from build123d import *

# Parameters (mm, degrees)
SKETCH_1_R        = 3
SKETCH_1_R_2      = 1.5
EXTRUDE_1_DEPTH   = 1.2
EXTRUDE_1_2_DEPTH = 1.2
EXTRUDE_2_DEPTH   = 1.2
FILLET_1_R        = 1


with BuildPart() as part:
    # Sketch 1 → Extrude 1 (new body)
    with BuildSketch(Plane.XY):
        with Locations((-4.672939719, 0.001012373)):
            Circle(SKETCH_1_R)
        with Locations((-4.672939719, 0.001012373)):
            Circle(SKETCH_1_R_2, mode=Mode.SUBTRACT)
    extrude(amount=EXTRUDE_1_DEPTH)



with BuildPart() as body_2:
    # Sketch 1 → Extrude 1 2 (new body)
    with BuildSketch(Plane.XY):
        with Locations((4.672939719, -0.001012373)):
            Circle(SKETCH_1_R)
        with Locations((4.672939719, -0.001012373)):
            Circle(SKETCH_1_R_2, mode=Mode.SUBTRACT)
    extrude(amount=EXTRUDE_1_2_DEPTH)


with BuildPart() as part_1:
    add(part.part)

    add(body_2.part)  # Extrude 2 merges body 2
    # Sketch 2 → Extrude 2 (add)
    with BuildSketch(Plane.XY.offset(1.2)):
        Polygon((-4.672103484, 3.001012257), (4.673403359, 2.998987591), (1.672939725, -0.001203708), (4.672476078, -3.001012337), (-4.673775953, -2.99898751), (-1.672939772, 0.001576302), align=None)
    extrude(amount=-EXTRUDE_2_DEPTH)

    # Fillet 1
    fillet_1_edges = [part_1.edges().sort_by_distance(p)[0] for p in [
        (3.172939719, -0.001012373, 1.2),
        (-6.172939719, 0.001012373, 1.2),
    ]]
    fillet(fillet_1_edges, radius=FILLET_1_R)


solid = part_1.part
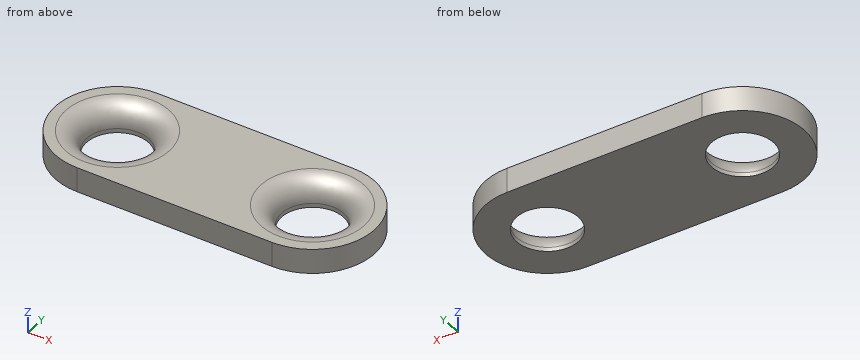
Source: CAD feature listing. Evaluate the final solid. Frame: model axes, mm. Round coordinates to 2 decimals unless told otherwise and drop trailing zeros. Loops run counter-clockwise (first coordinate to the right, second up) from the corner with the lowest first, then second, coordinate; pieces in that order, holes last. Notation, with made-up numbers: (0.5, 9.5) -> (13.5, 9.5) arc R23 ccw to (13.5, 38.5) -> close; hole circle Ø5 at (58.5, 1). An arc over 180 degrees is marked (long way). Answer as a JSON object with one key per item and string values. Group by question number.
Q1. Ray query, line 1 (X direction, y = 1.5, z = 0.9); line 2 (X direction, y = 0.5, z = 0.85); line 3 (Y direction, x = -2, z = 1.05). Return the intervals inside material, ascending. Write a range as from..to.
Q2. Contact query for a flat-ended pin moving along its axis: P1, Ø2.5, axis at x = -4.67, y = 0, coming from the -Z side. Output: stop coordinate, or through.
Q3. Section query B-B (y = 1). State how many separate pieces and enclosed holes the cut face has, plus the area to 3 significant figures.
Q4. Section query A-A (z = 0.65). Output: boundary loops of the cut face in (x, y), plus the area to 3 significant figures.
Completed:
{
 "1": {"line 1": "-7.27..-5.64, -3.7..3.71, 5.64..7.27", "line 2": "-7.63..-6.34, -3.01..3.01, 6.34..7.63", "line 3": "-3..3"},
 "2": {"P1": "through"},
 "3": {"separate pieces": "3", "enclosed holes": "0", "area": "11.6 mm²"},
 "4": {"outline": "(-4.67, -3) -> (4.67, -3) arc R3 ccw to (4.67, 3) -> (-4.67, 3) arc R3 ccw to start; hole circle Ø3.21 at (-4.67, 0); hole circle Ø3.21 at (4.67, 0)", "area": "68.1 mm²"}
}
